Verification items for the finished model (mm, model axes). A direction names the side the tool comes from. Coordinates: 2 decimals unless noted, no trailing zeros. Loops run counter-clockwise (first coordinate to the right, second up) from the corner with the lowest first, then second, coordinate; pieces in that order, holes last. Notation, with made-up numbers: (86, 71) - (118, 71) arc R19 cw to (118, 106) - close; hole circle Ø1 at (46, -39). An arc over 180 degrees is marked (long way). One line per item, written item: value. Start each with the question number.
(1) Section check B-B (y = 9). Record the boundary of the cut face in (x, z).
(2) Gauge pin test, flat ends, axial feed: P1, Ø1.5, axis at x = 31, z = 10, coming from the +Y side; P2, Ø10, axis at x = 65.5, z = 34, coming from the -Y side; P3, Ø1.5, axis at x = 52.5, z = 25.5, coming from the -Y side. Record the tip position at first contact, or that the pin passes through.
(3) Section check D-D (y = 18.5). Record the boundary of the cut face in (x, z).
(4) Section check A-A (z = 31). Record the boundary of the cut face in (x, y), plus the area to 3 significant figures.
(5) Thickness scan on probe 1 along Y at (x, z) = (-10, 70.5); probe 2 along X at (y, z) = (21.5, 5.5); probe 3 along Z at (x, y) = (32, 8.5). Record the ranges inside material, lowest first. Write a range as [from, to].
(6) Set-up check for faces 1 (the face through (28.63, 7.6, 66.46)), 2 (the face through (30, 15, 39)), 3 (the face through (8, 0, 39)), 4 (the face through (3.547, 22, 39)): record each of +Z, -Z, +X, -X, +Y, -Y from which the full face is reachable in a straight line by a thin tool's end or side.
(7) Draft check along Z on faces 5 (the face through (-12, 15, 39)), 6 (the face through (18, 9, 0)), 7 (the face through (68.838, -5.842, 53.986)). Enter one of: +Z half, -Z half, draft (parallel to the pull), parting line (faces both ways), or undercut.
(8) Section check C-C (x = 32). Record the boundary of the cut face in (y, z).
```python
from build123d import *

# Parameters (mm, degrees)
BOSS_EXTRUDE1_DEPTH = 80
FILLET1_R           = 40
SKETCH3_R           = 5
CUT_EXTRUDE3_DEPTH  = 15
SKETCH4_R           = 5
CUT_EXTRUDE4_DEPTH  = 80
SKETCH5_R           = 17.5
CUT_EXTRUDE5_DEPTH  = 26


with BuildPart() as part:
    # Sketch2 → Boss-Extrude1 (new body)
    with BuildSketch(Plane.XY):
        Polygon((-28.453333333, 0), (45.546666667, 0), (106.168444932, -35), (106.168444932, -20), (45.546666667, 15), (13.546666667, 15), (13.546666667, 28.653333333), (3.546666667, 28.653333333), (3.546666667, 15), (-28.453333333, 15), align=None)
    extrude(amount=BOSS_EXTRUDE1_DEPTH)

    # Fillet1
    # the kernel refuses this fillet: 40 mm, written as the material it takes off along each edge
    with BuildSketch(Plane(origin=(106.168444932, -135, 0), x_dir=(0, 0, 1), z_dir=(0, 1, 0))) as fillet1_piece_1:
        with BuildLine():
            CenterArc((FILLET1_R, -FILLET1_R), FILLET1_R, 90, 90)
            Line((0, -FILLET1_R), (0, 0))
            Line((0, 0), (FILLET1_R, 0))
        make_face()
    extrude(amount=215, mode=Mode.SUBTRACT)
    with BuildSketch(Plane(origin=(106.168444932, -135, 80), x_dir=(0, 0, -1), z_dir=(0, 1, 0))) as fillet1_piece_2:
        with BuildLine():
            CenterArc((FILLET1_R, FILLET1_R), FILLET1_R, 180, 90)
            Line((0, FILLET1_R), (0, 0))
            Line((0, 0), (FILLET1_R, 0))
        make_face()
    extrude(amount=215, mode=Mode.SUBTRACT)

    # Sketch3 → Cut-Extrude3 (cut)
    with BuildSketch(Plane(origin=(0, 0, 0), x_dir=(1, 0, 0), z_dir=(0, 1, 0))):
        with Locations(Location((-13.453333333, -19.550801078, 0), (0, 0, 90))):
            Circle(SKETCH3_R)
        with Locations(Location((-13.453333333, -62.802123194, 0), (0, 0, 90))):
            Circle(SKETCH3_R)
    extrude(amount=CUT_EXTRUDE3_DEPTH, mode=Mode.SUBTRACT)

    # Sketch4 → Cut-Extrude4 (cut)
    with BuildSketch(Plane(origin=(0, 15, 0), x_dir=(1, 0, 0), z_dir=(0, 1, 0))):
        with Locations(Location((30.546666667, -17.032746755, 0), (0, 0, 270))):
            Circle(SKETCH4_R)
        with Locations(Location((30.546666667, -61.843602222, 0), (0, 0, 270))):
            Circle(SKETCH4_R)
    extrude(amount=-CUT_EXTRUDE4_DEPTH, mode=Mode.SUBTRACT)

    # Sketch5 → Cut-Extrude5 (cut)
    with BuildSketch(Plane(origin=(17.881857195, 30.972285196, 0), x_dir=(0.866025403784438, -0.5000000000000011, 0), z_dir=(0.5000000000000011, 0.8660254037844382, 0))):
        with Locations(Location((71.944570391, -39.229988433, 0), (0, 0, 180))):
            Circle(SKETCH5_R)
    extrude(amount=-CUT_EXTRUDE5_DEPTH, mode=Mode.SUBTRACT)


solid = part.part
```
Responses:
1. outline: (-28.45, 0) - (55.94, 0) - (55.94, 80) - (-28.45, 80) - close; hole circle Ø10 at (-13.45, 19.55); hole circle Ø10 at (-13.45, 62.8); hole circle Ø10 at (30.55, 17.03); hole circle Ø10 at (30.55, 61.84)
2. P1: stops at y = 15
2. P2: stops at y = -6.54
2. P3: stops at y = -4.45
3. outline: (3.55, 0) - (13.55, 0) - (13.55, 80) - (3.55, 80) - close
4. outline: (-28.45, 0) - (45.55, 0) - (60.32, -8.53) - (66.81, 2.72) - (45.55, 15) - (13.55, 15) - (13.55, 28.65) - (3.55, 28.65) - (3.55, 15) - (-28.45, 15) - close; (87.07, -23.97) - (105.14, -34.41) - (105.14, -19.41) - (93.56, -12.72) - close
4. area: 1,740 mm²
5. probe 1: y = [0, 15]
5. probe 2: x = [3.55, 13.55]
5. probe 3: z = [0, 12.25], [21.82, 57.06], [66.63, 80]
6. face 1: +Y, -Y
6. face 2: +Z, -Z, +X, +Y
6. face 3: +Z, -Z, -X, -Y
6. face 4: +Z, -Z, -X, +Y
7. face 5: draft
7. face 6: -Z half
7. face 7: undercut
8. outline: (0, 0) - (15, 0) - (15, 12.25) - (0, 12.25) - close; (0, 21.82) - (15, 21.82) - (15, 57.06) - (0, 57.06) - close; (0, 66.63) - (15, 66.63) - (15, 80) - (0, 80) - close
